Source: CAD feature listing. Evaluate the final solid. Frame: model axes, mm. A direction names the side the tool comes from. Give positions to 0.01 mm unless a question says otherwise; leave off trailing zeros. Write each loop counter-clockwise with the first axis right and the second up, starting at its lowest first coordinate (ties: lowest second). Pieces come first, ordered by that corner, then holes. Notation, with made-up numbers: (84.25, 56) -> (136.25, 56) arc R21 cw to (136.25, 90) -> close; hole circle Ø10 at (-29, 11.5). An arc over 180 degrees is marked (long way). Use one line per item in the form item = value. Start each with the question number.
(1) Cut plane C-C, the plane z = 2.25. Count the separate pieces of the cut face and the enclosed holes in it, and give its area (3 significant figures).
(2) Cut plane D-D, the plane x = -3.5. Output: boundary loops of the cut face in (y, z) (3 decimals).
(3) Cut plane B-B, the plane z = 6.25. Output: boundary loops of the cut face in (x, y).
(4) First-contact query: P1, Ø1.5, axis at y = 47.5, z = 2.5, coming from the -X side; P2, Ø3, axis at x = -5.5, z = 6.5, coming from the -Y side; P3, Ø2, axis at x = -31.5, z = 1.5, coming from the +Y side; P4, Ø12, axis at x = -19.5, y = 7, coming from the +Z side. Flat tips, straight axial feed; report the tip coordinate or a pass-through.
(5) Cut plane A-A, the plane x = -12. Output: boundary loops of the cut face in (y, z) (3 decimals), and give its area (3 significant figures).
(6) Draft query along Y for faces 3 (the face through (-13.143, -3.086, 11.09)), 4 (the face through (-15.07, 62.41, 6.26)), 5 (the face through (-14.288, 15, 6)). Return one class per face: pulls with the +Y half, pulls with the -Y half, needs draft (parallel to the pull), parting line crosses it, or undercut.
(7) Set-up query: faces 1 (the face through (-11, 38, 0)), 2 (the face through (-7, -3, 9.525)). Return all of +Z, -Z, +X, -X, +Y, -Y with unobstructed straight access to the full face (end or side cutting, diameter ignored); none if empty.
(8) Material intervals for line 1 along X through (y, z) = (37.5, 5.75); line 2 along Y through (x, z) = (-34, 8); line 3 along Y through (x, z) = (-18, 6.25), sorted ascending. Write a range as from..to.
from build123d import *

# Parameters (mm, degrees)
SKETCH4_R           = 2.032
BOSS_EXTRUDE1_DEPTH = 12.7
SKETCH5_W           = 6.35
SKETCH5_H           = 6.47192
CUT_EXTRUDE1_DEPTH  = 15.2875
FILLET1_R           = 5.08


with BuildPart() as part:
    # Sketch4 → Boss-Extrude1 (new body)
    with BuildSketch(Plane.XY):
        with BuildLine():
            Line((0, -6.35), (-14.2875, -6.35))
            Line((-14.2875, -6.35), (-14.2875, 0))
            Line((-14.2875, 0), (-14.2875, 39.249775278))
            Line((-14.2875, 39.249775278), (-39.516769232, 69.316847523))
            ThreePointArc((-39.516769232, 69.316847523), (-38.636253228, 79.3811915), (-28.571909251, 78.500675497))
            Line((-28.571909251, 78.500675497), (0, 44.45))
            Line((0, 44.45), (0, 0))
            Line((0, 0), (0, -6.35))
        make_face()
        with Locations((-11.1125, -3.175)):
            Circle(SKETCH4_R, mode=Mode.SUBTRACT)
        with Locations((-3.175, -3.175)):
            Circle(SKETCH4_R, mode=Mode.SUBTRACT)
    extrude(amount=BOSS_EXTRUDE1_DEPTH)

    # Sketch5 → Cut-Extrude1 (cut, through all)
    with BuildSketch(Plane.ZY.offset(14.2875)):
        with Locations((6.35, -3.11404)):
            Rectangle(SKETCH5_W, SKETCH5_H)
    extrude(amount=-CUT_EXTRUDE1_DEPTH, mode=Mode.SUBTRACT)

    # Fillet1
    fillet1_edges = [part.edges().sort_by_distance(p)[0] for p in [
        (0, 44.45, 6.35),
        (-14.2875, 39.249775278, 6.35),
    ]]
    fillet(fillet1_edges, radius=FILLET1_R)


solid = part.part
Geometry says:
q1.separate_pieces = 1
q1.enclosed_holes = 2
q1.area = 1,340 mm^2
q2.outline = (-6.35, 0) -> (-5.181, 0) -> (-5.181, 3.175) -> (-6.35, 3.175) -> close; (-6.35, 9.525) -> (-5.181, 9.525) -> (-5.181, 12.7) -> (-6.35, 12.7) -> close; (-1.169, 0) -> (48.621, 0) -> (48.621, 12.7) -> (-1.169, 12.7) -> (-1.169, 9.525) -> (0.122, 9.525) -> (0.122, 3.175) -> (-1.169, 3.175) -> close
q3.outline = (-39.52, 69.32) -> (-15.48, 40.67) arc R5.08 cw to (-14.29, 37.4) -> (-14.29, 0.12) -> (0, 0.12) -> (0, 42.6) arc R5.08 ccw to (-1.19, 45.87) -> (-28.57, 78.5) arc R7.14 ccw to start
q4.P1 = -21.84
q4.P2 = 0.12
q4.P3 = 80.88
q4.P4 = 12.7
q5.outline = (-6.35, 0) -> (-5.003, 0) -> (-5.003, 3.175) -> (-6.35, 3.175) -> close; (-6.35, 9.525) -> (-5.003, 9.525) -> (-5.003, 12.7) -> (-6.35, 12.7) -> close; (-1.347, 0) -> (58.751, 0) -> (58.751, 12.7) -> (-1.347, 12.7) -> (-1.347, 9.525) -> (0.122, 9.525) -> (0.122, 3.175) -> (-1.347, 3.175) -> close
q5.area = 762 mm^2
q6.face_3 = undercut
q6.face_4 = pulls with the +Y half
q6.face_5 = needs draft
q7.face_1 = -Z, +X, -X, +Y, -Y
q7.face_2 = +X, -X, -Y
q8.line_1 = -14.29..0
q8.line_2 = 62.74..81.05
q8.line_3 = 43.67..65.9
